```python
from build123d import *

# Parameters (mm, degrees)
SKETCH2_R           = 2.55
BOSS_EXTRUDE1_DEPTH = 2.5
SKETCH3_R           = 11.5
SKETCH3_R_2         = 5.15
SKETCH3_R_3         = 1.75
BOSS_EXTRUDE2_DEPTH = 2.5


with BuildPart() as part:
    # Sketch2 → Boss-Extrude1 (new body)
    with BuildSketch(Plane(origin=(0, 0, 0), x_dir=(1, 0, 0), z_dir=(0, 1, 0))):
        with BuildLine():
            Line((0, 0), (0, -43.53))
            ThreePointArc((0, -43.53), (1.597239013, -49.511852877), (5.96376064, -53.901297623))
            Line((5.96376064, -53.901297623), (66.212357085, -88.966818103))
            ThreePointArc((66.212357085, -88.966818103), (72.562868254, -90.513731665), (78.730609731, -88.350193185))
            Line((78.730609731, -88.350193185), (86.683137673, -82.606205082))
            ThreePointArc((86.683137673, -82.606205082), (87.415064266, -80.369517058), (85.51209015, -78.984894595))
            Line((85.51209015, -78.984894595), (80.51209015, -78.984894595))
            ThreePointArc((80.51209015, -78.984894595), (79.097876588, -78.399108157), (78.51209015, -76.984894595))
            Line((78.51209015, -76.984894595), (78.51209015, -67.984894595))
            ThreePointArc((78.51209015, -67.984894595), (77.926303712, -66.570681032), (76.51209015, -65.984894595))
            Line((76.51209015, -65.984894595), (67.01209015, -65.984894595))
            ThreePointArc((67.01209015, -65.984894595), (65.597876588, -65.399108157), (65.01209015, -63.984894595))
            Line((65.01209015, -63.984894595), (65.01209015, -22.984894595))
            ThreePointArc((65.01209015, -22.984894595), (65.597876588, -21.570681032), (67.01209015, -20.984894595))
            Line((67.01209015, -20.984894595), (85.51209015, -20.984894595))
            ThreePointArc((85.51209015, -20.984894595), (86.926303712, -20.399108157), (87.51209015, -18.984894595))
            Line((87.51209015, -18.984894595), (87.51209015, -5.954894595))
            ThreePointArc((87.51209015, -5.954894595), (87.314017067, -5.087104652), (86.759030766, -4.391200539))
            Line((86.759030766, -4.391200539), (79.495671877, 1.400838623))
            ThreePointArc((79.495671877, 1.400838623), (72.762340359, 3.995319432), (65.758425997, 2.25915481))
            Line((65.758425997, 2.25915481), (63.980401456, 1.173012986))
            ThreePointArc((63.980401456, 1.173012986), (61.97611448, 0.29883463), (59.81, 0))
            Line((59.81, 0), (0, 0))
        make_face()
        with Locations(Location((71.997086471, -79.027657881, 0), (0, 0, 270))):
            Circle(SKETCH2_R, mode=Mode.SUBTRACT)
        with Locations(Location((11.9, -43.53, 0), (0, 0, 270))):
            Circle(SKETCH2_R, mode=Mode.SUBTRACT)
        with Locations(Location((31.6, -43.53, 0), (0, 0, 270))):
            Circle(SKETCH2_R, mode=Mode.SUBTRACT)
        with Locations(Location((57.6, -43.53, 0), (0, 0, 270))):
            Circle(SKETCH2_R, mode=Mode.SUBTRACT)
        with Locations(Location((72.11209015, -7.984894595, 0), (0, 0, 270))):
            Circle(SKETCH2_R, mode=Mode.SUBTRACT)
    extrude(amount=BOSS_EXTRUDE1_DEPTH)

    # Sketch3 → Boss-Extrude2 (add)
    with BuildSketch(Plane.XY):
        with BuildLine():
            Line((0, 2), (-1, 2))
            ThreePointArc((-1, 2), (-6.656854249, 4.343145751), (-9, 10))
            Line((-9, 10), (-9, 48.5))
            ThreePointArc((-9, 48.5), (-7.535533906, 52.035533906), (-4, 53.5))
            Line((-4, 53.5), (8.545082445, 53.5))
            Line((8.545082445, 53.5), (17.116766662, 53.5))
            Line((17.116766662, 53.5), (33.14, 53.5))
            ThreePointArc((33.14, 53.5), (35.733493255, 52.774785695), (37.574651147, 50.809517094))
            Line((37.574651147, 50.809517094), (62.964663137, 2.056534888))
            Line((62.964663137, 2.056534888), (0, 2))
        make_face()
        with Locations((12, 32.5)):
            Circle(SKETCH3_R, mode=Mode.SUBTRACT)
        with Locations((40.884663137, 17.186715743)):
            Circle(SKETCH3_R_2, mode=Mode.SUBTRACT)
        with Locations((40.884663137, 26.186715743)):
            Circle(SKETCH3_R_3, mode=Mode.SUBTRACT)
        with Locations((40.884663137, 8.186715743)):
            Circle(SKETCH3_R_3, mode=Mode.SUBTRACT)
        with Locations((-3.5, 48)):
            Circle(SKETCH3_R_3, mode=Mode.SUBTRACT)
        with Locations((27.313284257, 48)):
            Circle(SKETCH3_R_3, mode=Mode.SUBTRACT)
        with Locations((27.313284257, 17.186715743)):
            Circle(SKETCH3_R_3, mode=Mode.SUBTRACT)
        with Locations((-3.5, 17.186715743)):
            Circle(SKETCH3_R_3, mode=Mode.SUBTRACT)
    extrude(amount=BOSS_EXTRUDE2_DEPTH)


solid = part.part
```
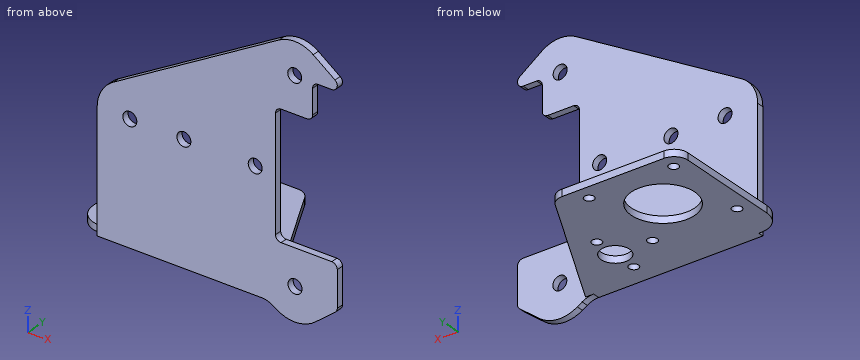
Can you work these out from the model? Positions are in its coordinate system, mm. Coordinates: 2 decimals unless noted, no trailing zeros. Write each loop counter-clockwise with the first axis right and the second up, starting at its lowest first coordinate (ties: lowest second). Pieces come first, ordered by that corner, then holes. Notation, with made-up numbers: M 50,15 L 97,15 A9 ccw 97,21 Z; hole C 3,-17.5 d8. An arc over 180 degrees is marked long. Write item = value, one per line. Start each with the question number.
Q1. If I drill on L1, parallel to Y at x = 53.5, z = 5.5, over which ranges is the centre line in solid material (lowest first)? Write a range as [from, to].
Q2. If we section it at D-D, the plane x = 41: Write out the boundary of the cut face in (y, z), then the cut area to 3 significant figures.
Q3. If we section it at C-C, the plane x = 57.6: Write out the boundary of the cut face in (y, z).
Q4. If we section it at B-B, the plane y = 32.5: Write out the boundary of the cut face in (x, z).
Q5. I'm going to push flat-ended pins straight in: pin 1 (5.5 mm diameter, centred on x = -3.5, y = 17.19, fed in from -Z); pin 2 (8 mm diameter, centred on x = 11.9, z = 43.53, fed in from +Y); pin 3 (3 mm diameter, centred on x = 71, y = 1.5, fed in from -Z); pin 4 (4 mm diameter, centred on x = 27.31, y = 48, fed in from +Z). Where does each tip first touch, or does it pass through?
Q6. If we section it at A-A, the plane x = 11.9: Write out the boundary of the cut face in (y, z), then the cut area to 3 significant figures.
Check sheet entries:
q1.L1 = [0, 2.5]
q2.outline = M 0,0 L 6.44,0 L 6.44,2.5 L 2.5,2.5 L 2.5,74.29 L 0,74.29 Z; M 9.93,0 L 12.04,0 L 12.04,2.5 L 9.93,2.5 Z; M 22.34,0 L 24.44,0 L 24.44,2.5 L 22.34,2.5 Z; M 27.93,0 L 44.23,0 L 44.23,2.5 L 27.93,2.5 Z
q2.area = 247 mm²
q3.outline = M 0,0 L 12.36,0 L 12.36,2.5 L 2.5,2.5 L 2.5,40.98 L 0,40.98 Z; M 0,46.08 L 2.5,46.08 L 2.5,83.95 L 0,83.95 Z
q4.outline = M -9,0 L 0.5,0 L 0.5,2.5 L -9,2.5 Z; M 23.5,0 L 47.11,0 L 47.11,2.5 L 23.5,2.5 Z
q5.pin_1 = 0
q5.pin_2 = 2.5
q5.pin_3 = -4.02
q5.pin_4 = 2.5
q6.outline = M 0,0 L 21,0 L 21,2.5 L 2.5,2.5 L 2.5,40.98 L 0,40.98 Z; M 0,46.08 L 2.5,46.08 L 2.5,57.36 L 0,57.36 Z; M 44,0 L 53.5,0 L 53.5,2.5 L 44,2.5 Z
q6.area = 201 mm²
